```python
from build123d import *

# Parameters (mm, degrees)
BOSS_EXTRUDE12_DEPTH            = 80
CUT_EXTRUDE10_DEPTH             = 80.5
CUT_EXTRUDE10_DEPTH_BACK        = 15.5
SKETCH37_W                      = 102
SKETCH37_H                      = 56
BOSS_EXTRUDE16_DEPTH            = 3
CUT_EXTRUDE11_DEPTH             = 86.294722428
SKETCH40_W                      = 127.486838651
SKETCH40_H                      = 54.833163407
CUT_EXTRUDE12_DEPTH             = 35.662124955
CUT_EXTRUDE12_DEPTH_BACK        = 1.75
CUT_EXTRUDE14_DEPTH             = 18.5
F_1_4_0_25_DIAMETER_HOLE1_D     = 6.35
F_1_4_0_25_DIAMETER_HOLE1_DEPTH = 5
F_1_4_0_25_DIAMETER_HOLE1_TIP   = 1.907732465
CHAMFER2_SIZE                   = 12
CHAMFER3_SIZE                   = 2
BOSS_EXTRUDE17_START            = -29
SKETCH50_W                      = 65
SKETCH50_H                      = 2
BOSS_EXTRUDE17_DEPTH            = 29
F_3_0MM_DOWEL_HOLE1_D           = 3
F_3_0MM_DOWEL_HOLE1_DEPTH       = 2


with BuildPart() as part:
    # Sketch22 → Boss-Extrude12 (new body)
    with BuildSketch(Plane.XY):
        with BuildLine():
            Line((32.5, -14.5), (-32.5, -14.5))
            ThreePointArc((-32.5, -14.5), (-47, 0), (-32.5, 14.5))
            Line((-32.5, 14.5), (32.5, 14.5))
            ThreePointArc((32.5, 14.5), (47, 0), (32.5, -14.5))
        make_face()
    extrude(amount=BOSS_EXTRUDE12_DEPTH)

    # Sketch35 → Cut-Extrude10 (cut, two sides)
    with BuildSketch(Plane(origin=(-32.5, 0, 0), x_dir=(0, 0, -1), z_dir=(1, 0, 0))) as cut_extrude10_sk:
        Polygon((0, 14.5), (-29.026860374, -14.5), (0, -14.5), align=None)
    extrude(amount=CUT_EXTRUDE10_DEPTH, mode=Mode.SUBTRACT)
    extrude(cut_extrude10_sk.sketch, amount=-CUT_EXTRUDE10_DEPTH_BACK, mode=Mode.SUBTRACT)

    # Sketch37 → Boss-Extrude16 (add)
    with BuildSketch(Plane(origin=(0, 7.256711984, 7.249996893), x_dir=(-1, 0, 0), z_dir=(0, -0.707434022, -0.706779389))):
        with Locations((0, -10.26729429)):
            Rectangle(SKETCH37_W, SKETCH37_H)
    extrude(amount=-BOSS_EXTRUDE16_DEPTH)

    # Sketch38 → Cut-Extrude11 (cut, through all)
    with BuildSketch(Plane.XY.offset(80)):
        with BuildLine():
            Line((-32.5, 12.75), (32.5, 12.75))
            ThreePointArc((32.5, 12.75), (45.25, 0), (32.5, -12.75))
            Line((32.5, -12.75), (-32.5, -12.75))
            ThreePointArc((-32.5, -12.75), (-45.25, 0), (-32.5, 12.75))
        make_face()
    extrude(amount=-CUT_EXTRUDE11_DEPTH, mode=Mode.SUBTRACT)

    # Sketch40 → Cut-Extrude12 (cut, two sides)
    with BuildSketch(Plane(origin=(0, -12.75, 0), x_dir=(1, 0, 0), z_dir=(0, 1, 0))) as cut_extrude12_sk:
        with Locations((5.984726224, -62.441589639)):
            Rectangle(SKETCH40_W, SKETCH40_H)
    extrude(amount=CUT_EXTRUDE12_DEPTH, mode=Mode.SUBTRACT)
    extrude(cut_extrude12_sk.sketch, amount=-CUT_EXTRUDE12_DEPTH_BACK, mode=Mode.SUBTRACT)

    # Sketch42 → Cut-Extrude14 (cut)
    with BuildSketch(Plane.ZY.offset(51)):
        Polygon((35.025007935, 14.5), (27.025007935, 14.5), (27.025007935, -8.259321849), (33.271466325, -14.5), (35.025007935, -14.5), align=None)
    extrude(amount=-CUT_EXTRUDE14_DEPTH, mode=Mode.SUBTRACT)

    # 1/4 (0.25) Diameter Hole1
    with Locations(Plane(origin=(0, 14.5, 0), x_dir=(1, 0, 0), z_dir=(0, 1, 0))):
        with Locations((2.6293e-05, -24.875007935)):
            Hole(F_1_4_0_25_DIAMETER_HOLE1_D / 2, depth=F_1_4_0_25_DIAMETER_HOLE1_DEPTH)
            with Locations((0, 0, -(F_1_4_0_25_DIAMETER_HOLE1_DEPTH + F_1_4_0_25_DIAMETER_HOLE1_TIP / 2))):  # 118° drill point
                Cone(0, F_1_4_0_25_DIAMETER_HOLE1_D / 2, F_1_4_0_25_DIAMETER_HOLE1_TIP, mode=Mode.SUBTRACT)

    # Chamfer2
    chamfer2_edges = [part.edges().sort_by_distance(p)[0] for p in [
        (51, -18.728671856, 35.381751886),
        (51, 20.850973922, -4.234553344),
        (-51, 20.850973922, -4.234553344),
        (-51, -18.728671856, 35.381751886),
    ]]
    chamfer(chamfer2_edges, length=CHAMFER2_SIZE)

    # Chamfer3
    chamfer3_edges = [part.edges().sort_by_distance(p)[0] for p in [
        (-51, 0, 14.513430187),
        (51, 0, 14.513430187),
        (0, -19.789822889, 34.321582802),
        (0, 19.789822889, -5.294722428),
        (-45, -15.549146556, 30.07697867),
        (45, -15.549146556, 30.07697867),
        (45, 15.549146556, -1.050118296),
        (-45, 15.549146556, -1.050118296),
    ]]
    chamfer(chamfer3_edges, length=CHAMFER3_SIZE)

    # Sketch50 → Boss-Extrude17 (add)
    with BuildSketch(Plane(origin=(0, 14.5, 0), x_dir=(1, 0, 0), z_dir=(0, 1, 0)).offset(BOSS_EXTRUDE17_START)):
        with Locations((0, -36.025007935)):
            Rectangle(SKETCH50_W, SKETCH50_H)
    extrude(amount=BOSS_EXTRUDE17_DEPTH)

    # Ø3.0mm Dowel Hole1
    with Locations(Plane(origin=(0, 0, 35.025007935), x_dir=(-1, 0, 0), z_dir=(0, 0, -1))):
        with Locations((-22.500026293, 0.25), (22.499973707, 0.25)):
            Hole(F_3_0MM_DOWEL_HOLE1_D / 2, depth=F_3_0MM_DOWEL_HOLE1_DEPTH)


solid = part.part
```
The listing builds one solid part. Answer for the finished solid, in the listing's coordinates (mm). A direction names the side the tool comes from. Round coordinates to 2 decimals unless told otherwise and drop trailing zeros. Loops run counter-clockwise (first coordinate to the right, second up) from the corner with the lowest first, then second, coordinate; pieces in that order, holes last. Notation, with made-up numbers: (88.25, 12.5) - (132.25, 12.5) arc R22 ccw to (132.25, 22.5) - close; hole circle Ø6 at (8.25, 38). An arc over 180 degrees is marked (long way). Use one line per item in the form item = value. Start each with the question number.
1. The part is cut by section B-B on z = 9. Determine the outline of the cut face in (x, y), then the cut area to 3 significant figures.
2. The part is cut by section A-A on x = -10. Determine the outline of the cut face in (y, z) (3 decimals), then the cut area to 3 significant figures.
3. For a pull along Y with two mould halves and no side action, classify faces 4 (the face through (0, -12.75, 31)), 5 (the face through (0, -14.5, 35)), 6 (the face through (49.99, 0.54, 15.37)), 7 (the face through (0, 14.5, 20)) as pulls with the +Y half, pulls with the -Y half, needs draft (parallel to the pull), parting line crosses it, or undercut.
4. A tool of negligible diameter and unlimited length cuts with its end or side. For faces 1 (the face through (46, 1, 35.025)), 2 (the face through (-44, 6, 27.025)), 3 (the face through (-50.014, 0.559, 15.389)), from which of +Z, -Z, +X, -X, +Y, -Y can it reach the whole face along a straight path? Write none if from no direction.
5. Given pin 1 Ø16.5 at (x, z) = (12, 20.5) entering from -Y; pin 2 Ø5 at (x, y) = (22.5, 0.25) entering from -Z (3 decimals); pin 3 Ø16.5 at (x, z) = (-9, 18.5) entering from +Y, each flat-ended and moving along its own axis, determine where each tip first touches the part or whether it passes through.
6. Consider line 1 (X direction, y = 0, z = 36); line 2 (Z direction, x = -9.5, y = -6) (3 decimals); line 3 (X direction, y = 3, z = 16). Determine where each line is inside the solid, lowest interval first. Write a range as [from, to].
7. The part is cut by section C-C on y = 0.25. Determine the outline of the cut face in (x, z) (3 decimals).
Geometry check:
q1.outline = (-51, 8.34) - (-49, 5.51) - (-44, 5.51) arc R12.75 cw to (-32.5, 12.75) - (32.5, 12.75) arc R12.75 cw to (44, 5.51) - (49, 5.51) - (51, 8.34) - (51, 9.75) - (43.23, 9.75) arc R14.5 ccw to (32.5, 14.5) - (-32.5, 14.5) arc R14.5 ccw to (-43.23, 9.75) - (-51, 9.75) - close
q1.area = 216 mm^2
q2.outline = (-18.376, 32.907) - (-12.75, 27.275) - (-12.75, 35.025) - (12.75, 35.025) - (12.75, 1.752) - (18.376, -3.88) - (21.205, -3.881) - (21.912, -3.174) - (14.5, 4.245) - (14.5, 37.025) - (-14.5, 37.025) - (-14.5, 33.271) - (-17.668, 36.442) - (-18.375, 35.735) - close
q2.area = 171 mm^2
q3.face_4 = undercut
q3.face_5 = undercut
q3.face_6 = pulls with the -Y half
q3.face_7 = pulls with the +Y half
q4.face_1 = +Z, +X, +Y
q4.face_2 = +Z, -X, +Y
q4.face_3 = -Z, -X, -Y
q5.pin_1 = -14.22
q5.pin_2 = 35.025
q5.pin_3 = 14.5
q6.line_1 = [-32.5, -23.98], [-21.02, 21.02], [23.98, 32.5]
q6.line_2 = [35.025, 37.025]
q6.line_3 = [-46.69, -44.89], [44.89, 46.69]
q7.outline = (-51, 17.093) - (-49, 14.263) - (-45.248, 14.263) - (-45.248, 27.025) - (-46.998, 27.025) - (-46.998, 18.508) - (-51, 18.508) - close; (-32.5, 35.025) - (-24, 35.025) - (-24, 37.025) - (-32.5, 37.025) - close; (-21, 35.025) - (21, 35.025) - (21, 37.025) - (-21, 37.025) - close; (24, 35.025) - (32.5, 35.025) - (32.5, 37.025) - (24, 37.025) - close; (45.248, 14.263) - (49, 14.263) - (51, 17.093) - (51, 18.508) - (46.998, 18.508) - (46.998, 35.025) - (45.248, 35.025) - close
